Part model, mm, in its own coordinate system. Face numbers are marked on the shaded views. A direction names the side the tool comes from. Coordinates: 2 decimals unless noted, no trailing zeros. Use one line per item in the form item = value. Start each with the question number.
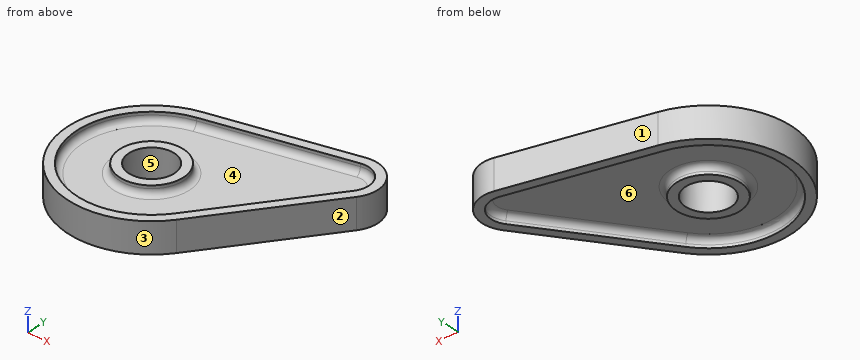
from build123d import *

# Parameters (mm, degrees)
SKETCH2_R           = 7.5
BOSS_EXTRUDE1_DEPTH = 10
SKETCH3_R           = 10.5
CUT_EXTRUDE1_DEPTH  = 3
CUT_EXTRUDE2_START  = -3
SKETCH4_R           = 10.5
CUT_EXTRUDE2_DEPTH  = 3
FILLET1_R           = 2


with BuildPart() as part:
    # Sketch2 → Boss-Extrude1 (new body)
    with BuildSketch(Plane.XY.offset(13)):
        with BuildLine():
            Line((-20.832934418, 37.628991133), (-66.388883934, 26.747563666))
            ThreePointArc((-66.388883934, 26.747563666), (-82.819662857, -15.34643239), (-37.637352066, -16.005060993))
            Line((-37.637352066, -16.005060993), (-10.377831921, 22.082582166))
            ThreePointArc((-10.377831921, 22.082582166), (-10.211644676, 33.483125214), (-20.832934418, 37.628991133))
        make_face()
        with Locations((-60, 0)):
            Circle(SKETCH2_R, mode=Mode.SUBTRACT)
    extrude(amount=BOSS_EXTRUDE1_DEPTH)

    # Sketch3 → Cut-Extrude1 (cut)
    with BuildSketch(Plane.XY.offset(23)):
        with BuildLine():
            Line((-20.135965261, 34.711075097), (-65.691914777, 23.82964763))
            ThreePointArc((-65.691914777, 23.82964763), (-80.330245091, -13.672276129), (-40.076913659, -14.25905434))
            Line((-40.076913659, -14.25905434), (-12.817393513, 23.82858882))
            ThreePointArc((-12.817393513, 23.82858882), (-12.701062442, 31.808968954), (-20.135965261, 34.711075097))
        make_face()
        with Locations((-60, 0)):
            Circle(SKETCH3_R, mode=Mode.SUBTRACT)
    extrude(amount=-CUT_EXTRUDE1_DEPTH, mode=Mode.SUBTRACT)

    # Sketch4 → Cut-Extrude2 (cut)
    with BuildSketch(Plane(origin=(0, 0, 13), x_dir=(-1, 0, 0), z_dir=(0, 0, -1)).offset(CUT_EXTRUDE2_START)):
        with BuildLine():
            Line((65.691914777, 23.82964763), (20.135965261, 34.711075097))
            ThreePointArc((20.135965261, 34.711075097), (12.701062442, 31.808968954), (12.817393513, 23.82858882))
            Line((12.817393513, 23.82858882), (40.076913659, -14.25905434))
            ThreePointArc((40.076913659, -14.25905434), (80.330245091, -13.672276129), (65.691914777, 23.82964763))
        make_face()
        with Locations(Location((60, 0, 0), (0, 0, 180))):
            Circle(SKETCH4_R, mode=Mode.SUBTRACT)
    extrude(amount=CUT_EXTRUDE2_DEPTH, mode=Mode.SUBTRACT)

    # Fillet1
    fillet1_edges = [part.edges().sort_by_distance(p)[0] for p in [
        (-42.913940019, 29.270361363, 20),
        (-12.701062442, 31.808968954, 20),
        (-26.447153586, 4.78476724, 20),
        (-80.330245091, -13.672276129, 20),
        (-70.5, 0, 20),
        (-12.701062442, 31.808968954, 16),
        (-42.913940019, 29.270361363, 16),
        (-80.330245091, -13.672276129, 16),
        (-26.447153586, 4.78476724, 16),
        (-70.5, 0, 16),
    ]]
    fillet(fillet1_edges, radius=FILLET1_R)


solid = part.part
Q1. Which spindle directions (+Z, -Z, +X, -X, +Y, -Y) get a long thin tool onto all of the face, cutting with end or side? Do the marked faces 5 and 6. Say none if no direction does.
Q2. Pin check, flat tips, straight feed: P1, Ø16.5, axis at x = -43, y = 0.5, coming from the +Z side; P2, Ø6, axis at y = -20.5, z = 14.5, coming from the +X side; P3, Ø2, axis at x = -60, y = -15.5, coming from the +Z side; P4, Ø1, axis at y = 3, z = 15, coming from the +X side. Stop position of each tip, or through.
Q3. Drill centre lines: probe 1 along X at (y, z) = (1.5, 14.75); probe 2 along X at (y, z) = (-8, 21.25); probe 3 along Z at (x, y) = (-64, -12.5). Where is each one in solid material? Low to high.
Q4. Mould opens along X. For the marked faces 1, 2, 3 and 4 say: released by +X, released by -X, zero draft, split by the parting line, or undercut.
Solution:
q1.face_5 = +Z, -Z
q1.face_6 = -Z
q2.P1 = 23
q2.P2 = -38.79
q2.P3 = 20
q2.P4 = -23.68
q3.probe_1 = -87.46 to -84.31, -70.54 to -67.35, -52.65 to -49.46, -28.98 to -25.11
q3.probe_2 = -86.31 to -83, -67.02 to -52.98, -35.78 to -31.91
q3.probe_3 = 16 to 20
q4.face_1 = released by -X
q4.face_2 = released by +X
q4.face_3 = split by the parting line
q4.face_4 = undercut
